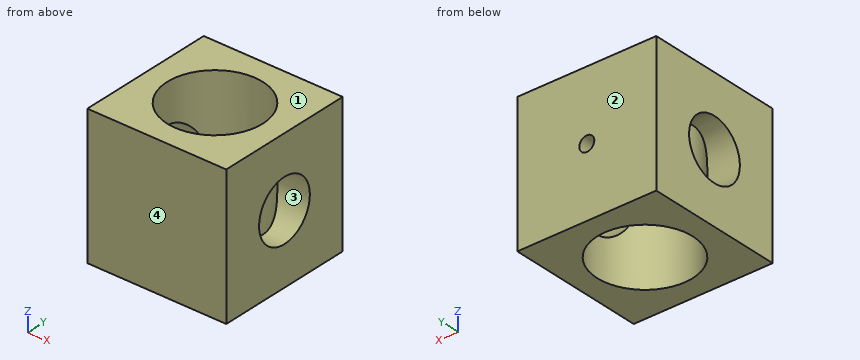
```python
from build123d import *

# Parameters (mm, degrees)
SKETCH3_W           = 25
SKETCH3_H           = 25
BOSS_EXTRUDE1_DEPTH = 25
CUT_EXTRUDE1_REACH  = 27
SKETCH4_R           = 8.6
CUT_EXTRUDE2_REACH  = 27
SKETCH5_R           = 1.35
SKETCH6_R           = 5.45
CUT_EXTRUDE3_DEPTH  = 26


with BuildPart() as part:
    # Sketch3 → Boss-Extrude1 (new body)
    with BuildSketch(Plane(origin=(0, 0, 0), x_dir=(1, 0, 0), z_dir=(0, 1, 0))):
        Rectangle(SKETCH3_W, SKETCH3_H)
    extrude(amount=BOSS_EXTRUDE1_DEPTH)

    # Sketch4 → Cut-Extrude1 (cut, up to next)
    with BuildSketch(Plane.XY.offset(12.5), mode=Mode.PRIVATE) as cut_extrude1_sk1:
        with Locations((0, 12.5)):
            Circle(SKETCH4_R)
    cut_extrude1_tool1 = extrude(cut_extrude1_sk1.sketch, amount=-CUT_EXTRUDE1_REACH, mode=Mode.PRIVATE) & part.part
    add(cut_extrude1_tool1.solids().sort_by_distance((0, 12.5, 12.5))[0], mode=Mode.SUBTRACT)

    # Sketch5 → Cut-Extrude2 (cut, up to next)
    with BuildSketch(Plane(origin=(0, 25, 0), x_dir=(1, 0, 0), z_dir=(0, 1, 0)), mode=Mode.PRIVATE) as cut_extrude2_sk1:
        Circle(SKETCH5_R)
    cut_extrude2_tool1 = extrude(cut_extrude2_sk1.sketch, amount=-CUT_EXTRUDE2_REACH, mode=Mode.PRIVATE) & part.part
    add(cut_extrude2_tool1.solids().sort_by_distance((0, 25, 0))[0], mode=Mode.SUBTRACT)

    # Sketch6 → Cut-Extrude3 (cut, through all)
    with BuildSketch(Plane.ZY.offset(12.5)):
        with Locations((0, 12.5)):
            Circle(SKETCH6_R)
    extrude(amount=-CUT_EXTRUDE3_DEPTH, mode=Mode.SUBTRACT)


solid = part.part
```
Model file for the job. Use its own axes, mm. Face numbers are marked on the shaded views. Coordinates: 2 decimals unless noted, no trailing zeros. Write each loop counter-clockwise with the first axis right and the second up, starting at its lowest first coordinate (ties: lowest second). Pieces come first, ordered by that corner, then holes. Notation, with made-up numbers: (-4.75, -29.75) - (24.25, -29.75) arc R19 ccw to (24.25, -13.75) - close; hole circle Ø1 at (43, 41). An arc over 180 degrees is marked (long way). Use a Markdown table: item, result. Add a question column.
Item 1: Two-plate mould, pull along Y, no slides. Class the marked faces 1, 2, 3 and 4: pulls with the +Y half, pulls with the -Y half, needs draft (parallel to the pull), parting line crosses it, or undercut.
Item 2: Band-saw the part on D-D, the plane x = 9.5. Write the cut outline in (y, z).
Item 3: Band-saw the part on A-A, the plane x = 0. Write the cut outline in (y, z), and give its area (3 significant figures).
Item 4: Drill centre lines: line 1 along X through (y, z) = (22.95, 0); line 2 along Y through (x, z) = (0, -7); line 3 along Y through (x, z) = (7.9, 0). Where is each one in solid material? Low to high.
Item 5: Band-saw the part on C-C, the plane z = -8.5. Write the cut outline in (x, y), and give its area (3 significant figures).
Item 6: Drop flat-ended pins along their axis: pin 1 (10.5 mm diameter, centred on x = 0, y = 12.5, fed in from -Z); pin 2 (2 mm diameter, centred on x = 0, z = 0, fed in from -Y). Give the stop position or say it passes through.
Item 7: Band-saw the part on B-B, the plane y = 12.5. Write the cut outline in (x, z), and give its area (3 significant figures).
A:
| question | item | result |
|---|---|---|
| 1 | face 1 | needs draft |
| 1 | face 2 | pulls with the +Y half |
| 1 | face 3 | undercut |
| 1 | face 4 | pulls with the -Y half |
| 2 | outline | (0, -12.5) - (25, -12.5) - (25, 12.5) - (0, 12.5) - close; hole circle Ø10.9 at (12.5, 0) |
| 3 | outline | (0, -12.5) - (3.9, -12.5) - (3.9, 12.5) - (0, 12.5) - close; (21.1, -12.5) - (25, -12.5) - (25, -1.35) - (21.1, -1.35) - close; (21.1, 1.35) - (25, 1.35) - (25, 12.5) - (21.1, 12.5) - close |
| 3 | area | 184 mm² |
| 4 | line 1 | x = -12.5 to -1.35, 1.35 to 12.5 |
| 4 | line 2 | y = 0 to 3.9, 21.1 to 25 |
| 4 | line 3 | y = 0 to 7.05, 17.95 to 25 |
| 5 | outline | (-12.5, 0) - (12.5, 0) - (12.5, 25) - (-12.5, 25) - close; hole circle Ø17.2 at (0, 12.5) |
| 5 | area | 393 mm² |
| 6 | pin 1 | passes through |
| 6 | pin 2 | stops at y = 0 |
| 7 | outline | (-12.5, -12.5) - (-8.6, -12.5) - (-8.6, -5.45) - (-12.5, -5.45) - close; (-12.5, 5.45) - (-8.6, 5.45) - (-8.6, 12.5) - (-12.5, 12.5) - close; (8.6, -12.5) - (12.5, -12.5) - (12.5, -5.45) - (8.6, -5.45) - close; (8.6, 5.45) - (12.5, 5.45) - (12.5, 12.5) - (8.6, 12.5) - close |
| 7 | area | 110 mm² |
